Autodesk Inventor part; units mm, degrees
ref_plane "YZ Plane" through (0, 0, 0) normal (1, 0, 0) x (0, 1, 0)
ref_plane "XZ Plane" through (0, 0, 0) normal (0, 1, 0) x (-1, 0, 0)
ref_plane "XY Plane" through (0, 0, 0) normal (0, 0, 1) x (1, 0, 0)
sketch "Эскиз1" plane through (0, 0, 0) normal (0, 0, 1) x (1, 0, 0)
  line L0 (0, 0) -> (-200, 0)
  line L1 (-200, 0) -> (-200, 10)
  line L2 (-200, 10) -> (0, 10)
  line L3 (0, 10) -> (0, 0)
  line L4 (-156.1916, 10) -> (-150.6349, 10) construction
  line L5 (-195, 10) -> (-188.1699, 3.1699)
  line L6 (-185, 10) -> (-178.1699, 3.1699)
  line L7 (-175, 10) -> (-168.1699, 3.1699)
  line L8 (-40, 10) -> (-34.5353, 10)
  line L9 (-30, 10) -> (-25, 10)
  line L10 (-23.8869, 10) -> (-18.8869, 10)
  line L11 (-45, 10) -> (-50, 10)
  line L12 (-200, 0) -> (-199, -1)
  line L13 (-200, 0) -> (-198.5858, 0) construction
  line L14 (-199, -1) -> (-199, 0)
  line L15 (-194, 0) -> (-194, -1)
  line L16 (-194, -1) -> (-193, 0)
  line L17 (0, 0) -> (-1, -1)
  line L18 (0, 0) -> (1.4142, 0) construction
  line L19 (-1, -1) -> (-1, 0)
  line L20 (-6, 0) -> (-6, -1)
  line L21 (-6, -1) -> (-7, 0)
  line L22 (-102, 0) -> (-102, -1)
  line L23 (-102, -1) -> (-103, 0)
  line L24 (-98, 0) -> (-98, -1)
  line L25 (-98, -1) -> (-97, 0)
  line L26 (-188.1699, 3.1699) -> (-190, 10)
  line L27 (-180, 10) -> (-178.1699, 3.1699)
  line L28 (-170, 10) -> (-168.1699, 3.1699)
  line L29 (-35, 10) -> (-41.8301, 3.1699)
  line L30 (-41.8301, 3.1699) -> (-40, 10)
  line L31 (-30, 10) -> (-31.8301, 3.1699)
  line L32 (-31.8301, 3.1699) -> (-25, 10)
  line L33 (-20, 10) -> (-21.8301, 3.1699)
  line L34 (-21.8301, 3.1699) -> (-15, 10)
  line L35 (-45, 10) -> (-51.8301, 3.1699)
  line L36 (-51.8301, 3.1699) -> (-50, 10)
  line L37 (-198, 0) -> (-200, 2)
  line L38 (-2, 0) -> (0, 2)
  point P0 (-200, 5)
  point P1 (-100, 0)
  point P2 (-191.5849, 6.5849)
  dimension "d0" = 200
  dimension "d1" = 10
  dimension "d3" = 45
  dimension "d4" = 5
  dimension "d7" = 5
  dimension "d8" = 45
  dimension "d9" = 45
  dimension "d10" = 0
  dimension "d11" = 0
  dimension "d21" = 45
  dimension "d22" = 45
  dimension "d23" = 1
  dimension "d25" = 1
  dimension "d26" = 135
  dimension "d27" = 1
  dimension "d29" = 1
  dimension "d30" = 45
  dimension "d31" = 2
  dimension "d32" = 45
  dimension "d33" = 1
  dimension "d34" = 1
  dimension "d35" = 2
  dimension "d36" = 45
  dimension "d37" = 75
  dimension "d38" = 5
  dimension "d40" = 5
  dimension "d41" = 5
  dimension "d42" = 5
  dimension "d43" = 150
  dimension "d44" = 5
  dimension "d46" = 5
  dimension "d47" = 5
  dimension "d48" = 5
  dimension "d49" = 5
  dimension "d51" = 45
  dimension "d52" = 75
  dimension "d53" = 5
  dimension "d54" = 5
  dimension "d55" = 75
  dimension "d56" = 75
  dimension "d57" = 45
  dimension "d58" = 45
  dimension "d59" = 45
  dimension "d60" = 75
  dimension "d67" = 45
  dimension "d68" = 2
  dimension "d69" = 4
  dimension "d70" = 45
  dimension "d71" = 2
  dimension "d72" = 4
extrude "Выдавливание1" add sketch "Эскиз1" along normal blind 4 contours L38 L0 L37 L1 L2 L5 L26 L6 L27 L7 L28 L36 L35 L30 L29 L31 L32 L33 L34 L3 | L20 L21 L0 | L16 L15 L0
fillet "Сопряжение1" radius 1 21 edges at (-190, 10, 2) (-188.1699, 3.1699, 2) (-195, 10, 2) (-185, 10, 2) (-178.1699, 3.1699, 2) (-180, 10, 2) (-168.1699, 3.1699, 2) (-175, 10, 2) (-170, 10, 2) (-50, 10, 2) (-51.8301, 3.1699, 2) (-41.8301, 3.1699, 2) (-31.8301, 3.1699, 2) (-30, 10, 2) (-40, 10, 2) (-45, 10, 2) (-35, 10, 2) (-25, 10, 2) (-20, 10, 2) (-21.8301, 3.1699, 2) (-15, 10, 2)
fillet "Сопряжение2" radius 1 2 edges at (0, 10, 2) (-200, 10, 2)
properties part number "trunk"
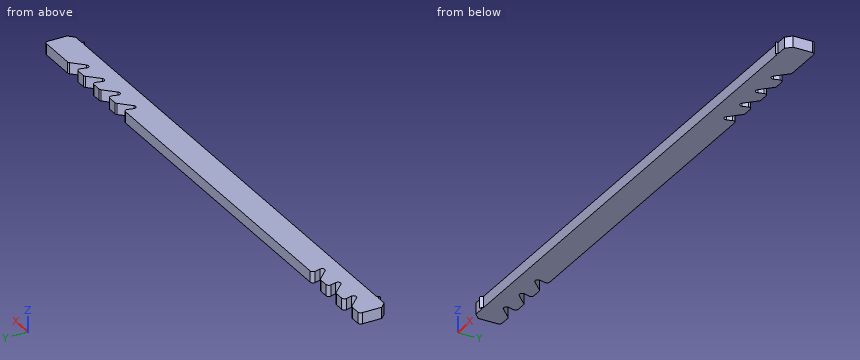
Geometry check sheet. Reference: the model listing, model coordinates, mm. Give positions to 0.01 mm unless a question says otherwise; leave off trailing zeros. Write each loop counter-clockwise with the first axis right and the second up, starting at its lowest first coordinate (ties: lowest second). Pieces come first, ordered by that corner, then holes.
1) Section check A-A, the plane x = -151. Record the boundary of the cut face in (y, z), and give its area (3 significant figures).
2) Material ranges on L1, parallel to Y at x = -55, z = 3.7; L2, parallel to Y at x = -16, z = 2, recorded low to high.
3) Gauge pin test, flat ends, axial feed: pin 1 (2 mm diameter, centred on x = -4.5, z = 2, fed in from -Y); pin 2 (0.5 mm diameter, centred on y = -0.5, z = 1.5, fed in from +X); pin 3 (4 mm diameter, centred on x = -69, y = 5.5, fed in from -Z); pin 4 (1.1 mm diameter, centred on y = -0.5, z = 2, fed in from -X). Record the tip position at first contact, or that the pin passes through.
4) Section check B-B, the plane x = -27.5. Record the boundary of the cut face in (y, z), and give its area (3 significant figures).
Computed:
1. outline: (0, 0) - (10, 0) - (10, 4) - (0, 4) - close
1. area: 40.0 mm2
2. L1: y = 0 to 10
2. L2: y = 0 to 9
3. pin 1: stops at y = 0
3. pin 2: stops at x = -6
3. pin 3: stops at z = 0
3. pin 4: stops at x = -198.05
4. outline: (0, 0) - (7.5, 0) - (7.5, 4) - (0, 4) - close
4. area: 30.0 mm2
